Can you work these out from the model? Positions are in its coordinate system, mm. A direction names the side the tool comes from. Give positions to 0.01 mm unless a question says otherwise; leave off trailing zeros. Order: outer loops, then holes, each group sorted by start corner. A loop starts at its lowest first (then second) coordinate and runs counter-clockwise, first axis right, second up.
Item 1: I want a section at B-B, the plane z = 15. Write out the boundary of the cut face in (x, y), then the cut area to 3 significant figures.
Item 2: If we mould it in two halves opening along X, with no side actions, what happens to faces 1 (the flat face through (0.99, 21.97, -49.98)), 2 (the flat face through (82, 2, -60)), 3 (the flat face through (67, 14, -59))? For each: +X half, -X half, draft (parallel to the pull), parting line (faces both ways), or undercut.
Item 3: I want a section at D-D, the plane z = 36. Write out the boundary of the cut face in (x, y), then the cut area to 3 significant figures.
Item 4: I want a section at C-C, the plane y = 10. Count the separate pieces of the cut face and the enclosed holes in it, then the cut area to 3 significant figures.
Item 5: I'm going to push flat-ended pins straight in: pin 1 Ø4 at (x, y) = (91, 49.5) entering from -Z; pin 2 Ø2 at (x, z) = (93.5, 33.5) entering from -Y; pin 3 Ø1.5 at (x, y) = (68, 6) entering from -Z; pin 4 Ø12 at (y, z) = (40, 25.5) entering from +X. Where does each tip first touch, or does it pass through?
Item 6: I want a section at A-A, the plane x = 27.5. Write out the boundary of the cut face in (y, z), then the cut area to 3 significant figures.
Item 7: Which directions (+Z, -Z, +X, -X, +Y, -Y) give clear straight access to the entire face, cutting with the end or side of a thin tool? Please do faces 4 (the flat face through (54, 10, 60)), 5 (the flat face through (94.01, 24.51, 49.14)), 6 (the flat face through (84, 3, 59)), 7 (the flat face through (44.72, 26.288, -52.811)).
Item 8: If I drill on line 1 along X through (y, z) = (51.1, -17.5); line 2 along Z through (x, y) = (27, 50); line 3 along X through (y, z) = (8.5, 57.5), over which ranges is the centre line in solid material (lowest first)?
```python
from build123d import *

# Parameters (mm, degrees)
EXTRUDE_1_DEPTH          = 95
EXTRUDE_3_DEPTH          = 20
CUT_EXTRUDE_1_DEPTH      = 142.209950074
CUT_EXTRUDE_1_DEPTH_BACK = 142.209950074
SKETCH_4_W               = 7
SKETCH_4_H               = 3
CUT_EXTRUDE_2_DEPTH      = 142.209950074
SHELL_START              = 2
SHELL_1_DEPTH            = 91
SHELL_START_2            = 93
SHELL_1_2_DEPTH          = 2.83772234
SHELL_1_3_DEPTH          = 3
CUT_EXTRUDE_3_DEPTH      = 3
SKETCH_7_R               = 1.75
SKETCH_7_W               = 10
SKETCH_7_H               = 50
CUT_EXTRUDE_4_DEPTH      = 142.209950074
SKETCH_9_W               = 15
SKETCH_9_H               = 20
CUT_EXTRUDE_5_DEPTH      = 3
EXTRUDE_4_DEPTH          = 2
EXTRUDE_6_DEPTH          = 2
SKETCH_13_W              = 40
SKETCH_13_H              = 28
CUT_EXTRUDE_6_DEPTH      = 2
CUT_EXTRUDE_7_DEPTH      = 10
FILLET_1_R               = 5
FILLET_2_R               = 5
EXTRUDE_7_DEPTH          = 2
EXTRUDE_8_DEPTH          = 2
SKETCH_17_R              = 1.75
EXTRUDE_9_DEPTH          = 2
SKETCH_18_W              = 120.1322677
SKETCH_18_H              = 134.585681159
CUT_EXTRUDE_8_DEPTH      = 2
SKETCH_20_W              = 175.540954957
SKETCH_20_H              = 97.306035525
CUT_EXTRUDE_9_DEPTH      = 39
CUT_EXTRUDE_10_DEPTH     = 39
SKETCH_23_W              = 6
SKETCH_23_H              = 5
SKETCH_23_W_2            = 3
SKETCH_23_H_2            = 3
CUT_EXTRUDE_11_DEPTH     = 181.790250578


with BuildPart() as part:
    # 草图1 → 凸台-拉伸1 (new body)
    with BuildSketch(Plane(origin=(0, 0, 0), x_dir=(0, 0, -1), z_dir=(1, 0, 0))):
        Polygon((-62.5, 0), (-45, 53), (45, 53), (62.5, 0), align=None)
    extrude(amount=EXTRUDE_1_DEPTH)

    # 草图3 → 凸台-拉伸3 (add)
    with BuildSketch(Plane(origin=(95, 0, 0), x_dir=(0, 0, -1), z_dir=(1, 0, 0))):
        Polygon((-60.849056604, 5), (-47.5, 5), (-47.5, 0), (-62.5, 0), align=None)
        Polygon((62.5, 0), (60.849056604, 5), (47.5, 5), (47.5, 0), align=None)
    extrude(amount=EXTRUDE_3_DEPTH)

    # 草图4 → 切除-拉伸1 (cut, two sides: drawn at the far end of the back side and taken through both)
    with BuildSketch(Plane.XY.offset(-CUT_EXTRUDE_1_DEPTH_BACK)):
        with Locations((105, 1.5)):
            Rectangle(SKETCH_4_W, SKETCH_4_H)
    extrude(amount=CUT_EXTRUDE_1_DEPTH + CUT_EXTRUDE_1_DEPTH_BACK, mode=Mode.SUBTRACT)

    # 草图5 → 切除-拉伸2 (cut, through all)
    with BuildSketch(Plane.XZ):
        with BuildLine():
            Line((97.5, -59), (97.5, -51))
            ThreePointArc((97.5, -51), (99, -49.5), (100.5, -51))
            Line((100.5, -51), (100.5, -59))
            ThreePointArc((100.5, -59), (99, -60.5), (97.5, -59))
        make_face()
        with BuildLine():
            Line((109.5, -59), (109.5, -51))
            ThreePointArc((109.5, -51), (111, -49.5), (112.5, -51))
            Line((112.5, -51), (112.5, -59))
            ThreePointArc((112.5, -59), (111, -60.5), (109.5, -59))
        make_face()
        with BuildLine():
            Line((97.5, 51), (97.5, 59))
            ThreePointArc((97.5, 59), (99, 60.5), (100.5, 59))
            Line((100.5, 59), (100.5, 51))
            ThreePointArc((100.5, 51), (99, 49.5), (97.5, 51))
        make_face()
        with BuildLine():
            Line((109.5, 51), (109.5, 59))
            ThreePointArc((109.5, 59), (111, 60.5), (112.5, 59))
            Line((112.5, 59), (112.5, 51))
            ThreePointArc((112.5, 51), (111, 49.5), (109.5, 51))
        make_face()
    extrude(amount=-CUT_EXTRUDE_2_DEPTH, mode=Mode.SUBTRACT)

    # 抽壳1: read off the stored shape, not the designer's step
    # 抽壳1 outline → 抽壳1 (cut)
    with BuildSketch(Plane.YZ.offset(SHELL_START)):
        Polygon((51, 43.554172654), (0, 60.393795296), (0, -60.393795296), (51, -43.554172654), align=None)
    extrude(amount=SHELL_1_DEPTH, mode=Mode.SUBTRACT)

    # Shell 1 2 outline → Shell 1 2 (cut)
    with BuildSketch(Plane.YZ.offset(SHELL_START_2)):
        Polygon((3, 49.5), (3, 59.403229258), (0, 60.393795296), (0, 49.5), align=None)
        Polygon((3, -49.5), (0, -49.5), (0, -60.393795296), (3, -59.403229258), align=None)
    extrude(amount=SHELL_1_2_DEPTH, mode=Mode.SUBTRACT)

    # Shell 1 3 outline → Shell 1 3 (add)
    with BuildSketch(Plane(origin=(0, 0, 0), x_dir=(1, 0, 0), z_dir=(0, 1, 0))):
        with BuildLine():
            Line((95.789496196, -60.393795296), (95.83772234, -60.504880632))
            Line((95.83772234, -60.504880632), (95.83772234, -49.5))
            ThreePointArc((95.83772234, -49.5), (95.585474278, -50.231225589), (95.5, -51))
            Line((95.5, -51), (95.5, -59))
            ThreePointArc((95.5, -59), (95.57313822, -59.711771272), (95.789496196, -60.393795296))
        make_face()
        with BuildLine():
            ThreePointArc((95.789496196, 60.393795296), (95.57313822, 59.711771272), (95.5, 59))
            Line((95.5, 59), (95.5, 51))
            ThreePointArc((95.5, 51), (95.585474278, 50.231225589), (95.83772234, 49.5))
            Line((95.83772234, 49.5), (95.83772234, 60.504880632))
            Line((95.83772234, 60.504880632), (95.789496196, 60.393795296))
        make_face()
    extrude(amount=SHELL_1_3_DEPTH)

    # 草图6 → 切除-拉伸3 (cut)
    with BuildSketch(Plane(origin=(95, 0, 0), x_dir=(0, 0, -1), z_dir=(1, 0, 0))):
        with BuildLine():
            Line((-37.770863272, 48), (37.770863272, 48))
            ThreePointArc((37.770863272, 48), (40.700157086, 47.052065862), (42.518739858, 44.567695099))
            Line((42.518739858, 44.567695099), (55.583544844, 5))
            Line((55.583544844, 5), (47.5, 5))
            Line((47.5, 5), (47.5, 0))
            Line((47.5, 0), (-47.5, 0))
            Line((-47.5, 0), (-47.5, 5))
            Line((-47.5, 5), (-55.583544844, 5))
            Line((-55.583544844, 5), (-42.518739858, 44.567695099))
            ThreePointArc((-42.518739858, 44.567695099), (-40.700157086, 47.052065862), (-37.770863272, 48))
        make_face()
    extrude(amount=-CUT_EXTRUDE_3_DEPTH, mode=Mode.SUBTRACT)

    # 草图7 → 切除-拉伸4 (cut, through all)
    with BuildSketch(Plane(origin=(0, 53, 0), x_dir=(1, 0, 0), z_dir=(0, 1, 0))):
        with Locations(Location((60, -15, 0), (0, 0, 270))):
            Circle(SKETCH_7_R)
        with Locations(Location((60, 17.5, 0), (0, 0, 270))):
            Circle(SKETCH_7_R)
        with Locations(Location((27.5, 17.5, 0), (0, 0, 270))):
            Circle(SKETCH_7_R)
        with Locations(Location((27.5, -15, 0), (0, 0, 270))):
            Circle(SKETCH_7_R)
        with Locations((90, 0)):
            Rectangle(SKETCH_7_W, SKETCH_7_H)
    extrude(amount=-CUT_EXTRUDE_4_DEPTH, mode=Mode.SUBTRACT)

    # 草图9 → 切除-拉伸5 (cut)
    with BuildSketch(Plane(origin=(0, 18.608057138, 56.35583019), x_dir=(1, 0, 0), z_dir=(0, 0.3135390198315126, 0.949575317204009))):
        with Locations((62.5, -9.596188739)):
            Rectangle(SKETCH_9_W, SKETCH_9_H)
    extrude(amount=-CUT_EXTRUDE_5_DEPTH, mode=Mode.SUBTRACT)

    # 草图10 → 凸台-拉伸4 (add)
    with BuildSketch(Plane(origin=(0, 18.608057138, 56.35583019), x_dir=(1, 0, 0), z_dir=(0, 0.3135390198315126, 0.949575317204009))):
        Polygon((55, -19.596188739), (54, -19.596188739), (54, 1.403811261), (71, 1.403811261), (71, -19.596188739), (70, -19.596188739), (70, 0.403811261), (55, 0.403811261), align=None)
    extrude(amount=EXTRUDE_4_DEPTH)

    # 草图11 → 凸台-拉伸6 (add)
    with BuildSketch(Plane(origin=(0, 18.608057138, -56.35583019), x_dir=(-1, 0, 0), z_dir=(0, 0.3135390198315126, -0.949575317204009))):
        Polygon((-67, -19.596188739), (-67, 10.403811261), (-23, 10.403811261), (-23, -19.596188739), (-25, -19.596188739), (-25, 8.403811261), (-65, 8.403811261), (-65, -19.596188739), align=None)
    extrude(amount=EXTRUDE_6_DEPTH)

    # 草图13 → 切除-拉伸6 (cut)
    with BuildSketch(Plane(origin=(0, 18.608057138, -56.35583019), x_dir=(-1, 0, 0), z_dir=(0, 0.3135390198315126, -0.949575317204009))):
        with Locations((-45, -5.596188739)):
            Rectangle(SKETCH_13_W, SKETCH_13_H)
    extrude(amount=-CUT_EXTRUDE_6_DEPTH, mode=Mode.SUBTRACT)

    # 草图14 → 切除-拉伸7 (cut)
    with BuildSketch(Plane.ZY):
        Polygon((-41.385431636, 48), (41.385431636, 48), (57.23448824, 0), (-57.23448824, 0), align=None)
    extrude(amount=-CUT_EXTRUDE_7_DEPTH, mode=Mode.SUBTRACT)

    # 圆角1
    fillet_1_edges = [part.edges().sort_by_distance(p)[0] for p in [
        (47.5, 53, 45),
        (47.5, 53, -45),
    ]]
    fillet(fillet_1_edges, radius=FILLET_1_R)

    # 圆角2
    fillet_2_edges = [part.edges().sort_by_distance(p)[0] for p in [
        (1, 48, -41.385431636),
        (1, 48, 41.385431636),
    ]]
    fillet(fillet_2_edges, radius=FILLET_2_R)

    # 草图15 → 凸台-拉伸7 (add)
    with BuildSketch(Plane(origin=(0, 17.980979099, 54.456679556), x_dir=(-1, 0, 0), z_dir=(0, -0.3135390198315126, -0.949575317204009))):
        with BuildLine():
            Line((-70, -18.935811381), (-70, 0.403811261))
            Line((-70, 0.403811261), (-55, 0.403811261))
            Line((-55, 0.403811261), (-55, -18.935811381))
            Line((-55, -18.935811381), (-2, -18.935811381))
            Line((-2, -18.935811381), (-2, 34.772408574))
            Line((-2, 34.772408574), (-93, 34.772408574))
            Line((-93, 34.772408574), (-93, -15.776504325))
            Line((-93, -15.776504325), (-95.523305282, -15.776504325))
            add(Edge.make_bspline(
                [(-95.789496196, -18.935811381), (-95.583035108, -17.41903761), (-95.523305282, -15.776504325)],
                knots=[1.16121292, 1.16121292, 1.16121292, 1.455331574, 1.455331574, 1.455331574], degree=2, weights=[1, 0.989206251, 1]))
            Line((-95.789496196, -18.935811381), (-70, -18.935811381))
        make_face()
    extrude(amount=EXTRUDE_7_DEPTH)

    # 草图16 → 凸台-拉伸8 (add)
    with BuildSketch(Plane(origin=(0, 17.980979099, -54.456679556), x_dir=(1, 0, 0), z_dir=(0, -0.3135390198315126, 0.949575317204009))):
        with BuildLine():
            Line((65, 8.403811261), (65, -18.935811381))
            Line((65, -18.935811381), (95.789496196, -18.935811381))
            add(Edge.make_bspline(
                [(95.523305282, -15.776504325), (95.583035108, -17.41903761), (95.789496196, -18.935811381)],
                knots=[4.827853734, 4.827853734, 4.827853734, 5.121972388, 5.121972388, 5.121972388], degree=2, weights=[1, 0.989206251, 1]))
            Line((95.523305282, -15.776504325), (93, -15.776504325))
            Line((93, -15.776504325), (93, 34.772408574))
            Line((93, 34.772408574), (2, 34.772408574))
            Line((2, 34.772408574), (2, -18.935811381))
            Line((2, -18.935811381), (25, -18.935811381))
            Line((25, -18.935811381), (25, 8.403811261))
            Line((25, 8.403811261), (65, 8.403811261))
        make_face()
    extrude(amount=EXTRUDE_8_DEPTH)

    # 草图17 → 凸台-拉伸9 (add)
    with BuildSketch(Plane.XZ.offset(-51)):
        Polygon((85, 25), (93, 25), (93, 43.554172654), (2, 43.554172654), (2, -43.554172654), (93, -43.554172654), (93, -25), (85, -25), align=None)
        with Locations(Location((60, -17.5, 0), (0, 0, 90))):
            Circle(SKETCH_17_R, mode=Mode.SUBTRACT)
        with Locations(Location((27.5, -17.5, 0), (0, 0, 90))):
            Circle(SKETCH_17_R, mode=Mode.SUBTRACT)
        with Locations(Location((60, 15, 0), (0, 0, 90))):
            Circle(SKETCH_17_R, mode=Mode.SUBTRACT)
        with Locations(Location((27.5, 15, 0), (0, 0, 90))):
            Circle(SKETCH_17_R, mode=Mode.SUBTRACT)
    extrude(amount=EXTRUDE_9_DEPTH)

    # 草图18 → 切除-拉伸8 (cut)
    with BuildSketch(Plane(origin=(0, 0, 0), x_dir=(1, 0, 0), z_dir=(0, 1, 0))):
        with Locations((58.156973339, 0.12316308)):
            Rectangle(SKETCH_18_W, SKETCH_18_H)
    extrude(amount=-CUT_EXTRUDE_8_DEPTH, mode=Mode.SUBTRACT)

    # 草图20 → 切除-拉伸9 (cut)
    with BuildSketch(Plane(origin=(95, 0, 0), x_dir=(0, 0, -1), z_dir=(1, 0, 0))):
        with Locations((3.171805167, 26.174924158)):
            Rectangle(SKETCH_20_W, SKETCH_20_H)
    extrude(amount=CUT_EXTRUDE_9_DEPTH, mode=Mode.SUBTRACT)

    # 草图21 → 切除-拉伸10 (cut)
    with BuildSketch(Plane(origin=(95, 0, 0), x_dir=(0, 0, -1), z_dir=(1, 0, 0))):
        Polygon((-43.861204642, 40.501944611), (-57.23448824, 0), (57.23448824, 0), (43.861204642, 40.501944611), align=None)
    extrude(amount=-CUT_EXTRUDE_10_DEPTH, mode=Mode.SUBTRACT)

    # 草图23 → 切除-拉伸11 (cut, through all)
    with BuildSketch(Plane.XY.offset(-80)):
        with Locations((92, 2.5)):
            Rectangle(SKETCH_23_W, SKETCH_23_H)
        with Locations((82.5, 3.5)):
            Rectangle(SKETCH_23_W_2, SKETCH_23_H_2)
    extrude(amount=CUT_EXTRUDE_11_DEPTH, mode=Mode.SUBTRACT)


solid = part.part
```
Results list:
1. outline: (0, 48) - (2, 48) - (2, 49) - (25.75, 49) - (25.75, 53) - (0, 53) - close; (29.25, 49) - (58.25, 49) - (58.25, 53) - (29.25, 53) - close; (61.75, 49) - (85, 49) - (85, 53) - (61.75, 53) - close
1. area: 314 mm2
2. face 1: draft
2. face 2: undercut
2. face 3: +X half
3. outline: (0, 48) - (2, 48) - (2, 49) - (93, 49) - (93, 48) - (95, 48) - (95, 53) - (0, 53) - close
3. area: 384 mm2
4. separate pieces: 4
4. enclosed holes: 0
4. area: 590 mm2
5. pin 1: stops at z = -46.82
5. pin 2: stops at y = 48
5. pin 3: stops at z = -60.77
5. pin 4: passes through
6. outline: (0, 58.29) - (49, 42.11) - (49, 16.75) - (53, 16.75) - (53, 41.39) arc R5 ccw to (49.57, 46.13) - (0, 62.5) - close; (25.33, -49.92) - (27.22, -55.62) - (29.11, -54.99) - (28.49, -53.09) - (49.57, -46.13) arc R5 ccw to (53, -41.39) - (53, -19.25) - (49, -19.25) - (49, -42.11) - close; (49, -15.75) - (53, -15.75) - (53, 13.25) - (49, 13.25) - close
6. area: 640 mm2
7. face 4: +Z, -X, +Y
7. face 5: +X, -X, -Y
7. face 6: +Z, -Z
7. face 7: -Z, -Y
8. line 1: x = 0 to 25.75, 29.25 to 58.25, 61.75 to 85
8. line 2: z = -45.97 to -19.18, -15.82 to 13.32, 16.68 to 45.97
8. line 3: x = 0 to 55, 70 to 95
